from build123d import *

# Parameters (mm, degrees)
SKIZZE2_R                       = 1.5
AUFSATZ_LINEAR_AUSTRAGEN1_DEPTH = 5.5
SKIZZE3_W                       = 2.75
SKIZZE3_H                       = 3
SCHNITT_LINEAR_AUSTRAGEN1_DEPTH = 1.5
KREISMUSTER1_COUNT              = 5
SKIZZE4_R                       = 1.6
SCHNITT_LINEAR_AUSTRAGEN5_DEPTH = 37.075926877
SKIZZE5_R                       = 8
SCHNITT_LINEAR_AUSTRAGEN6_DEPTH = 13
VERRUNDUNG1_R                   = 1


with BuildPart() as part:
    # Skizze1 → Rotation1 (revolve)
    with BuildSketch(Plane.XY, mode=Mode.PRIVATE) as rotation1_sk:
        Polygon((0, 0), (6, 0), (6, 7.15), (8, 7.15), (8, 0), (19.5, 0), (19.5, -9.35), (0, -9.35), align=None)
    revolve(rotation1_sk.sketch.rotate(Axis((19.5, -9.35, 0), (-1, 0, 0)), 90), axis=Axis((19.5, -9.35, 0), (-1, 0, 0)))

    # Skizze2 → Aufsatz-Linear austragen1 (add)
    with BuildSketch(Plane.ZY.offset(-19.5)):
        with Locations((0, -5.35)):
            Circle(SKIZZE2_R)
    aufsatz_linear_austragen1 = extrude(amount=-AUFSATZ_LINEAR_AUSTRAGEN1_DEPTH)

    # Skizze3 → Schnitt-Linear austragen1 (cut)
    with BuildSketch(Plane(origin=(0, -3.85, 0), x_dir=(1, 0, 0), z_dir=(0, 1, 0))):
        with Locations((23.625, 0)):
            Rectangle(SKIZZE3_W, SKIZZE3_H)
    schnitt_linear_austragen1 = extrude(amount=-SCHNITT_LINEAR_AUSTRAGEN1_DEPTH, mode=Mode.SUBTRACT)

    # Kreismuster1: Aufsatz-Linear austragen1, Schnitt-Linear austragen1 ×5 about axis
    kreismuster1_axis = Axis((0, -9.35, 0), (1, 0, 0))
    add([aufsatz_linear_austragen1.rotate(kreismuster1_axis, i * 360 / KREISMUSTER1_COUNT) for i in range(1, KREISMUSTER1_COUNT)])
    add([schnitt_linear_austragen1.rotate(kreismuster1_axis, i * 360 / KREISMUSTER1_COUNT) for i in range(1, KREISMUSTER1_COUNT)], mode=Mode.SUBTRACT)

    # Skizze4 → Schnitt-Linear austragen5 (cut, through all)
    with BuildSketch(Plane(origin=(6, 0, 0), x_dir=(0, 0, -1), z_dir=(1, 0, 0))):
        with Locations((0, 3.4)):
            Circle(SKIZZE4_R)
        with Locations((11.041823898, -15.725)):
            Circle(SKIZZE4_R)
        with Locations((-11.041823898, -15.725)):
            Circle(SKIZZE4_R)
    extrude(amount=SCHNITT_LINEAR_AUSTRAGEN5_DEPTH, mode=Mode.SUBTRACT)

    # Skizze5 → Schnitt-Linear austragen6 (cut)
    with BuildSketch(Plane.ZY):
        with Locations((0, -9.35)):
            Circle(SKIZZE5_R)
    extrude(amount=-SCHNITT_LINEAR_AUSTRAGEN6_DEPTH, mode=Mode.SUBTRACT)

    # Verrundung1
    verrundung1_edges = [part.edges().sort_by_distance(p)[0] for p in [
        (19.5, -9.35, 9.35),
    ]]
    fillet(verrundung1_edges, radius=VERRUNDUNG1_R)


solid = part.part
Geometry check sheet. Reference: the model listing, model coordinates, mm. A direction names the side the tool comes from. Round coordinates to 2 decimals unless told otherwise and drop trailing zeros. Loops run counter-clockwise (first coordinate to the right, second up) from the corner with the lowest first, then second, coordinate; pieces in that order, holes last.
Item 1: Mould release check, pull along Y, two halves, no side actions. Record for faces 1 (the flat face through (23.61, -12.57, 2.37)), 2 (the cylindrical face through (6.986, -15.244, 9.516)), 3 (the flat face through (25, -8, 3)), 4 (the cylindrical face through (21.6, -7.867, -2.325)): pulls with the +Y half, pulls with the -Y half, needs draft (parallel to the pull), parting line crosses it, or undercut.
Item 2: Gauge pin test, flat ends, axial feed: pin 1 (1.4 mm diameter, centred on x = 24, z = -0.5, fed in from +Y); pin 2 (2 mm diameter, centred on y = -8, z = -5, fed in from +X); pin 3 (3 mm diameter, centred on x = 16.5, z = -3, fed in from +Y). Record the tip position at first contact, or that the pin passes through.
Item 3: Cross-section at A-A on z = 0. Record the boundary of the cut face in (x, y).
Item 4: Cross-section at C-C on x = 16.75. Record the boundary of the cut face in (y, z), then the cut area to 3 significant figures.
Item 5: Cross-section at D-D on y = 5.5. Record the boundary of the cut face in (x, z), then the cut area to 3 significant figures.
Item 6: Access from +Z, -Z, +X, -X, +Y, -Y to the whole of each face (thin tool, end or side, straight path). Record for faces 5 (the flat face through (22.25, -8, 4)), 6 (the cylindrical face through (21.6, -8.26, 2.31)), 7 (the flat face through (23.6, -8.1, -3.8)).
Item 7: Thickness scan on line 1 (Y direction, x = 7.35, z = 0); line 2 (Y direction, x = 9, z = 0); line 3 (X direction, y = -7.5, z = -4). Record the ranges inside material, lowest first.
Item 8: Cross-section at B-B on x = 3. Record the boundary of the cut face in (y, z).
Answer sheet:
1. face 1: pulls with the -Y half
1. face 2: undercut
1. face 3: needs draft
1. face 4: undercut
2. pin 1: stops at y = -5.35
2. pin 2: stops at x = 22.25
2. pin 3: stops at y = -0.12
3. outline: (0, -18.7) - (6, -18.7) - (6, -25.85) - (8, -25.85) - (8, -18.7) - (18.5, -18.7) arc R1 ccw to (19.5, -17.7) - (19.5, -6.85) - (25, -6.85) - (25, -5.35) - (22.25, -5.35) - (22.25, -3.85) - (19.5, -3.85) - (19.5, -1) arc R1 ccw to (18.5, 0) - (8, 0) - (8, 1.8) - (6, 1.8) - (6, 0) - (0, 0) - (0, -1.35) - (13, -1.35) - (13, -17.35) - (0, -17.35) - close; (6, 5) - (8, 5) - (8, 7.15) - (6, 7.15) - close
4. outline: circle Ø18.7 at (-9.35, 0)
4. area: 275 mm2
5. outline: (6, -7.19) - (8, -7.19) - (8, 7.19) - (6, 7.19) - close
5. area: 28.8 mm2
6. face 5: +Z, +X, +Y
6. face 6: +X
6. face 7: -Z, +X, +Y
7. line 1: y = -25.85 to -17.35, -1.35 to 1.8, 5 to 7.15
7. line 2: y = -18.7 to -17.35, -1.35 to 0
7. line 3: x = 13 to 22.25
8. outline: circle Ø18.7 at (-9.35, 0); hole circle Ø16 at (-9.35, 0)
